```python
from build123d import *

# Parameters (mm, degrees)
F0_W     = 384
F0_H     = 406
F2_DEPTH = 6
F3_D     = 3.4
F5_D     = 3.4
F4_R     = 75
F6_DEPTH = 6
F8_D     = 3.4
F9_D     = 3.4
F10_D    = 3.4


# Not quite as in the source:
# - a feature names something its author has since deleted; it is built from what else it names


with BuildPart() as f2:
    # F0 (on Front) → F2 (new body)
    with BuildSketch(Plane.XZ):
        Rectangle(F0_W, F0_H)
    extrude(amount=F2_DEPTH)

    # F3 (through all)
    with Locations(Plane(origin=(0, 0, 0), x_dir=(1, 0, 0), z_dir=(0, 1, 0))):
        with Locations((189, -150), (189, -50), (189, 150), (150, 200), (-50, 200), (-150, 200), (-189, -50), (-189, -150), (-189, 50)):
            Hole(F3_D / 2)

    # F5 (through all)
    with Locations(Plane(origin=(0, 0, 0), x_dir=(-1, 0, 0), z_dir=(0, 1, 0))):
        with Locations((98.3422863406, 48), (20.4, -87), (-57.5422863406, 48), (98.3422863406, -42), (20.4, 93), (-57.5422863406, -42)):
            Hole(F5_D / 2)


with BuildPart() as f6:
    # F4 (on face) → F6 (new body)
    with BuildSketch(Plane(origin=(0, 0, 0), x_dir=(-1, 0, 0), z_dir=(0, 1, 0))):
        with Locations((20.4, 3)):
            Circle(F4_R)
    extrude(amount=-F6_DEPTH)


with BuildPart() as f2_1:
    add(f2.part)

    # F7: cut F6
    add(f6.part, mode=Mode.SUBTRACT)

    # F8 (through all)
    with Locations(Plane(origin=(0, 0, 0), x_dir=(1, 0, 0), z_dir=(0, 1, 0))):
        with Locations((-189, 150)):
            Hole(F8_D / 2)

    # F9 (through all)
    with Locations(Plane(origin=(0, 0, 0), x_dir=(1, 0, 0), z_dir=(0, 1, 0))):
        with Locations((189, 50)):
            Hole(F9_D / 2)

    # F10 (through all)
    with Locations(Plane(origin=(0, 0, 0), x_dir=(1, 0, 0), z_dir=(0, 1, 0))):
        with Locations((50, 200)):
            Hole(F10_D / 2)


solid = f2_1.part
```
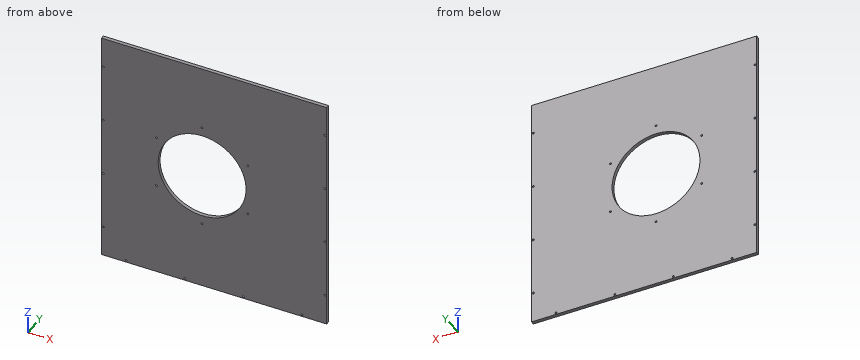
CAD build for the part. Positions are in the model's coordinates, mm. Round coordinates to 2 decimals unless told otherwise and drop trailing zeros. Loops run counter-clockwise (first coordinate to the right, second up) from the corner with the lowest first, then second, coordinate; pieces in that order, holes last. Notation, with made-up numbers: M 43.25,-26 L 91.25,-26 A25 cw 91.25,-10 Z; hole C -13.75,5 d8. An arc over 180 degrees is marked long. Use a Markdown table: item, result. Add a question column.
(1) Flat gauge pin, fed straight in: pin 1 (3 mm diameter, centred on x = 57.54, z = -42, fed in from -Y). Where does the tip first touch, or does it go through?
(2) Cut at A-A (y = -1.8). State how many separate pieces and enclosed holes the cut face has, and give its area (3 significant figures).
(3) Drill centre lines: line 1 (X direction, y = -2.65, z = -200); line 2 (X direction, y = -1.35, z = -87); line 3 (X direction, y = -4.8, z = 150). Where is each one in solid material? Low to high.
(4) Cut at C-C (z = -15). Give the cut face in (x, y), and give its area (3 significant figures).
(5) Cut at B-B (x = -63). Give the cut face in (y, z), and give its area (3 significant figures).
Geometry says:
| question | item | result |
|---|---|---|
| 1 | pin 1 | passes through |
| 2 | separate pieces | 1 |
| 2 | enclosed holes | 19 |
| 2 | area | 138,000 mm² |
| 3 | line 1 | x = -192 to -151.7, -148.3 to -51.7, -48.3 to 48.3, 51.7 to 148.3, 151.7 to 192 |
| 3 | line 2 | x = -192 to -22.1, -18.7 to 192 |
| 3 | line 3 | x = -192 to -190.7, -187.3 to 187.3, 190.7 to 192 |
| 4 | outline | M -192,-6 L -93.21,-6 L -93.21,0 L -192,0 Z; M 52.41,-6 L 192,-6 L 192,0 L 52.41,0 Z |
| 4 | area | 1,430 mm² |
| 5 | outline | M -6,-203 L 0,-203 L 0,-58.73 L -6,-58.73 Z; M -6,64.73 L 0,64.73 L 0,203 L -6,203 Z |
| 5 | area | 1,700 mm² |
